Autodesk Inventor part; units mm, degrees
ref_plane "YZ Plane" through (0, 0, 0) normal (1, 0, 0) x (0, 1, 0)
ref_plane "XZ Plane" through (0, 0, 0) normal (0, 1, 0) x (-1, 0, 0)
ref_plane "XY Plane" through (0, 0, 0) normal (0, 0, 1) x (1, 0, 0)
sketch "Sketch1" plane through (0, 0, 0) normal (0, 1, 0) x (-1, 0, 0)
  line L0 (704.85, 816.737) -> (-704.85, 816.737)
  line L1 (-704.85, 816.737) -> (-704.85, -816.737)
  line L2 (-704.85, -816.737) -> (704.85, -816.737)
  line L3 (704.85, -816.737) -> (704.85, 816.737)
  line L4 (704.85, 816.737) -> (-704.85, -816.737) construction
  line L5 (-704.85, 816.737) -> (704.85, -816.737) construction
  line L6 (692.15, 804.037) -> (-692.15, 804.037)
  line L7 (-692.15, 804.037) -> (-692.15, -804.037)
  line L8 (-692.15, -804.037) -> (692.15, -804.037)
  line L9 (692.15, -804.037) -> (692.15, 804.037)
  line L10 (692.15, 804.037) -> (-692.15, -804.037) construction
  line L11 (-692.15, 804.037) -> (692.15, -804.037) construction
  point P0 (0, 0)
  dimension "d0" = 1409.7
  dimension "d1" = 1633.474
  dimension "d2" = 12.7
  dimension "d3" = 12.7
extrude "Extrusion1" add sketch "Sketch1" along normal blind 1397
properties part number "AM14U3-gameVolume" material "Polycarbonate, Clear"
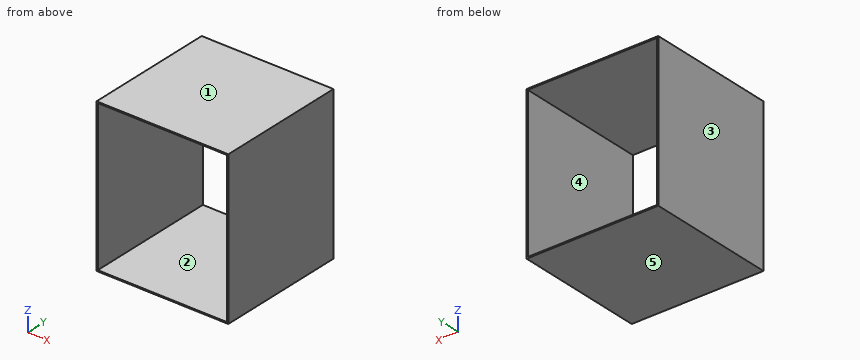
Can you work these out from the model? Positions are in its coordinate system, mm. Face numbers are marked on the shaded views. A direction names the side the tool comes from. Round coordinates to 2 decimals unless told otherwise and drop trailing zeros. Order: outer loops, then holes, each group sorted by start corner. A loop starts at its lowest first (then second) coordinate and runs counter-clockwise, first axis right, second up. Notation, with made-up numbers: (52, 26) -> (107, 26) arc R37 ccw to (107, 64) -> close; hole circle Ø5 at (10.5, 53.25). An arc over 180 degrees is marked (long way). Return JSON: item names as keys, results as strings. Group by question number.
1. If we section it at B-B, the plane x = -253.5: Write out the boundary of the cut face in (y, z).
2. Which directions (+Z, -Z, +X, -X, +Y, -Y) give clear straight access to the entire face, cutting with the end or side of a thin tool? Please do the marked faces 1 and 2.
3. We'd pull the mould along Z, two halves only. Please class the marked faces 3, 4 and 5: released by +Z, released by -Z, zero draft, split by the parting line, or undercut.
4. If we section it at A-A, the plane z = 356.5: Write out the boundary of the cut face in (x, y).
5. If we section it at C-C, the plane y = 1127: Write out the boundary of the cut face in (x, z), then the cut area to 3 significant figures.
6. I need wall thicknesses on line 1 (Z direction, x = -350, y = 782.5); line 2 (X direction, y = 958.5, z = 741). Which ranges of each line are inside material? Lowest first, please. Write a range as [from, to].
Output values:
{
 "1": {"outline": "(0, -816.74) -> (1397, -816.74) -> (1397, -804.04) -> (0, -804.04) -> close; (0, 804.04) -> (1397, 804.04) -> (1397, 816.74) -> (0, 816.74) -> close"},
 "2": {"face 1": "+Z, +X, -X, +Y, -Y", "face 2": "+Y, -Y"},
 "3": {"face 3": "zero draft", "face 4": "undercut", "face 5": "released by -Z"},
 "4": {"outline": "(-704.85, 0) -> (-692.15, 0) -> (-692.15, 1397) -> (-704.85, 1397) -> close; (692.15, 0) -> (704.85, 0) -> (704.85, 1397) -> (692.15, 1397) -> close"},
 "5": {"outline": "(-704.85, -816.74) -> (704.85, -816.74) -> (704.85, 816.74) -> (-704.85, 816.74) -> close; hole (-692.15, -804.04) -> (692.15, -804.04) -> (692.15, 804.04) -> (-692.15, 804.04) -> close", "area": "76,700 mm²"},
 "6": {"line 1": "[-816.74, -804.04], [804.04, 816.74]", "line 2": "[-704.85, -692.15], [692.15, 704.85]"}
}
